Can you work these out from the drawing? Everything is in mm from the part's minimum corner. A direction names the side the tool comes from. Round coordinates to 2 decimals unless told otherwise and drop trailing zeros. Loops run counter-clockwise (first coordinate to the right, second up) from the corner with the lowest first, then second, coordinate; pieces in that order, holes last. Notation, with made-up numbers: (-30, 29.5) -> (15, 29.5) arc R26 ccw to (15, 59.5) -> close; hole circle Ø2 at (47.5, 4.5). An arc over 180 degrees is marked (long way). One line per item, written item: value.
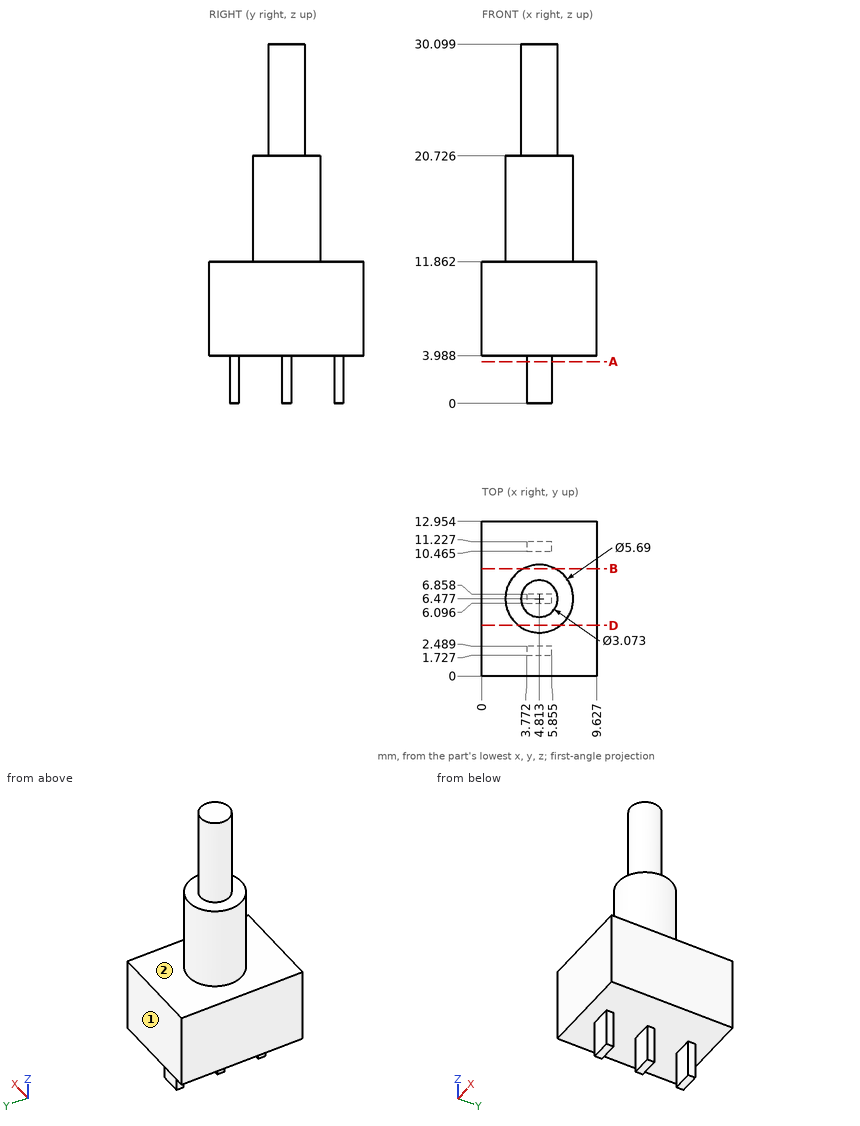
(1) Please list where these lines run through material, in increasing order: L1, parallel to Z at x = 2.25, y = 4.25; L2, parallel to Z at x = 7, y = 5; L3, parallel to X at y = 6.5, z = 15.
Results below:
L1: z = 3.99 to 11.86
L2: z = 3.99 to 20.73
L3: x = 1.97 to 7.66
(2) Imagine slicing it at D-D on y = 4.25. Write out the boundary of the cut face in (x, z).
Results below:
outline: (0, 3.99) -> (9.63, 3.99) -> (9.63, 11.86) -> (6.58, 11.86) -> (6.58, 20.73) -> (3.04, 20.73) -> (3.04, 11.86) -> (0, 11.86) -> close
(3) Imagine slicing it at A-A on z = 3.5. Write out the boundary of the cut face in (x, y) (1 decimal).
Results below:
outline: (3.8, 1.7) -> (5.9, 1.7) -> (5.9, 2.5) -> (3.8, 2.5) -> close; (3.8, 6.1) -> (5.9, 6.1) -> (5.9, 6.9) -> (3.8, 6.9) -> close; (3.8, 10.5) -> (5.9, 10.5) -> (5.9, 11.2) -> (3.8, 11.2) -> close
(4) On a 3-axis mill with a long thin cutter (end or side, diameter ignored), from which of +Z, -Z, +X, -X, +Y, -Y can I reach the whole of each face in a straight line? I mean the marked faces 1 and 2. Say none if no direction works.
Results below:
face 1: +Z, -Z, +X, -X, +Y
face 2: +Z
(5) Imagine slicing it at B-B on y = 9. Write out the boundary of the cut face in (x, z).
Results below:
outline: (0, 3.99) -> (9.63, 3.99) -> (9.63, 11.86) -> (6.13, 11.86) -> (6.13, 20.73) -> (3.5, 20.73) -> (3.5, 11.86) -> (0, 11.86) -> close
(6) For pin 1 Ø2.5 at (x, z) = (5, 2) entering from -Y; pin 2 Ø0.8 at (y, z) = (10.5, 1.5) entering from -X; pin 3 Ø0.8 at (y, z) = (2, 2.5) entering from +X (1 decimal), each with a flat end and sliding along its axis, tell me the tip position at first contact or that it passes through.
Results below:
pin 1: stops at y = 1.73
pin 2: stops at x = 3.77
pin 3: stops at x = 5.9
